Input: part model. Units: mm. Frame: model coordinates. Face numbers are marked on the shaded views. A direction names the side the tool comes from. Coordinates: 2 decimals unless noted, no trailing zeros. Loops run counter-clockwise (first coordinate to the right, second up) from the corner with the lowest first, then second, coordinate; pieces in that order, holes last. Notation, with made-up numbers: (6, 48) -> (51, 48) arc R14 cw to (51, 73) -> close; hole circle Ø6 at (51, 6). An arc over 180 degrees is marked (long way). Answer as a JSON object with one key per item and string values.
from build123d import *

# Parameters (mm, degrees)
SKETCH1_W               = 60
SKETCH1_H               = 10
BOSS_EXTRUDE1_DEPTH     = 150
CUT_EXTRUDE3_DEPTH      = 154.05227865
CUT_EXTRUDE3_DEPTH_BACK = 50
FILLET5_R               = 3
FILLET6_R               = 3
FILLET7_R               = 3


with BuildPart() as part:
    # Sketch1 → Boss-Extrude1 (new body)
    with BuildSketch(Plane.XY):
        Rectangle(SKETCH1_W, SKETCH1_H)
    extrude(amount=BOSS_EXTRUDE1_DEPTH)

    # Sketch2 → Cut-Extrude3 (cut, two sides: drawn at the far end of the back side and taken through both)
    with BuildSketch(Plane(origin=(0, 0, 0), x_dir=(-1, 0, 0), z_dir=(0, 0, -1)).offset(-CUT_EXTRUDE3_DEPTH_BACK)):
        Polygon((-30, 5), (-30, -5), (0, 5), align=None)
    extrude(amount=CUT_EXTRUDE3_DEPTH + CUT_EXTRUDE3_DEPTH_BACK, mode=Mode.SUBTRACT)

    # Fillet5
    fillet5_edges = [part.edges().sort_by_distance(p)[0] for p in [
        (15, 5, 50),
        (30, 0, 50),
        (-15, 5, 0),
    ]]
    fillet(fillet5_edges, radius=FILLET5_R)

    # Fillet6
    fillet6_edges = [part.edges().sort_by_distance(p)[0] for p in [
        (-30, -1.5, 0),
        (-30, 4.121320344, 0.878679656),
        (-30, 5, 76.5),
    ]]
    fillet(fillet6_edges, radius=FILLET6_R)

    # Fillet7
    # the kernel refuses this fillet: 3 mm, written as the material it takes off along each edge
    with BuildSketch(Plane(origin=(27, 2, 53), x_dir=(1, 0, 0), z_dir=(0, 1, 0))) as fillet7_piece_1_section:
        Polygon((0, 0), (FILLET7_R, 0), (FILLET7_R, FILLET7_R), (0, FILLET7_R), align=None)
    fillet7_piece_1 = extrude(amount=FILLET7_R, mode=Mode.PRIVATE)
    fillet7_piece_1 = fillet7_piece_1 - Plane(origin=(27, 2, 53), x_dir=(-0.7071067811865475, 0, 0.7071067811865475), z_dir=(0, 1, 0)) * Sphere(FILLET7_R, mode=Mode.PRIVATE)
    add(fillet7_piece_1, mode=Mode.SUBTRACT)
    with BuildSketch(Plane(origin=(30, 5, 53), x_dir=(-1, 0, 0), z_dir=(0, 0, 1))) as fillet7_piece_2:
        with BuildLine():
            CenterArc((FILLET7_R, FILLET7_R), FILLET7_R, 180, 90)
            Line((0, FILLET7_R), (0, 0))
            Line((0, 0), (FILLET7_R, 0))
        make_face()
    extrude(amount=104.5, mode=Mode.SUBTRACT)


solid = part.part
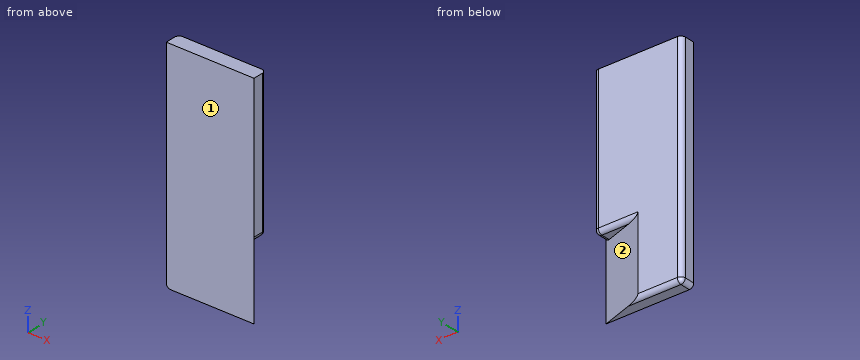
1. Section query B-B (z = 27). Return loops of the section in (x, y).
Reply:
{"outline": "(-30, -5) -> (30, -5) -> (0, 5) -> (-27, 5) arc R3 ccw to (-30, 2) -> close"}
2. Section query A-A (y = -0.75). Return loops of the section in (x, z).
Reply:
{"outline": "(-30, 3) arc R3 ccw to (-27, 0) -> (17.25, 0) -> (17.25, 50) -> (27, 50) arc R3 ccw to (30, 53) -> (30, 150) -> (-30, 150) -> close"}
3. Line query: line 1 along Z through (x, y) = (25.5, 1.5); line 2 along X through (y, z) = (2.5, 60.5); line 3 along X through (y, z) = (4.25, 92). Output: solid intervals per line, ascending.
Reply:
{"line 1": "z = 50 to 150", "line 2": "x = -29.96 to 29.96", "line 3": "x = -28.98 to 28.98"}
4. Access query for the marked faces 1 and 2. Directions: +Z, -Z, +X, -X, +Y, -Y. A direction counts if a zero-diameter tool reaches every point of the face in a straight line with its end or side. Return the directions, or none.
Reply:
{"face 1": "+Z, -Z, +X, -X, -Y", "face 2": "-Z, +X, +Y"}
